Here's how the part is built. I have some questions about the finished solid (model axes, mm). Face numbers are marked on the shaded views. A direction names the side the tool comes from. Give positions to 0.01 mm unless a question says otherwise; leave off trailing zeros. Write each loop counter-clockwise with the first axis right and the second up, starting at its lowest first coordinate (ties: lowest second). Pieces come first, ordered by that corner, then holes. Notation, with made-up numbers: (-27.5, 53) -> (23.5, 53) arc R14 ccw to (23.5, 70) -> close; hole circle Ø3 at (82.5, 42). An arc over 180 degrees is marked (long way). Use one line per item in the form item = value.
```python
from build123d import *

# Parameters (mm, degrees)
SKETCH1_W           = 19
SKETCH1_H           = 19
BOSS_EXTRUDE1_DEPTH = 8
SKETCH2_R           = 1.75
CUT_EXTRUDE1_DEPTH  = 16.636495771
SKETCH3_W           = 6
SKETCH3_H           = 6
BOSS_EXTRUDE2_DEPTH = 12
FILLET1_R           = 2
SKETCH5_W           = 4
SKETCH5_H           = 4
BOSS_EXTRUDE4_DEPTH = 4
FILLET3_R           = 1


with BuildPart() as part:
    # Sketch1 → Boss-Extrude1 (new body)
    with BuildSketch(Plane(origin=(0, 0, 0), x_dir=(1, 0, 0), z_dir=(0, 1, 0))):
        Rectangle(SKETCH1_W, SKETCH1_H)
    extrude(amount=BOSS_EXTRUDE1_DEPTH)

    # Sketch2 → Cut-Extrude1 (cut, through all)
    with BuildSketch(Plane(origin=(0, 8, 0), x_dir=(1, 0, 0), z_dir=(0, 1, 0))):
        with Locations(Location((-6.5, 6.5, 0), (0, 0, 270))):
            Circle(SKETCH2_R)
        with Locations(Location((6.5, 6.5, 0), (0, 0, 270))):
            Circle(SKETCH2_R)
        with Locations(Location((-6.5, -6.5, 0), (0, 0, 270))):
            Circle(SKETCH2_R)
        with Locations(Location((6.5, -6.5, 0), (0, 0, 270))):
            Circle(SKETCH2_R)
    extrude(amount=-CUT_EXTRUDE1_DEPTH, mode=Mode.SUBTRACT)

    # Sketch3 → Boss-Extrude2 (add)
    with BuildSketch(Plane(origin=(0, 8, 0), x_dir=(1, 0, 0), z_dir=(0, 1, 0))):
        Rectangle(SKETCH3_W, SKETCH3_H)
    extrude(amount=BOSS_EXTRUDE2_DEPTH)

    # Fillet1
    fillet1_edges = [part.edges().sort_by_distance(p)[0] for p in [
        (-9.5, 4, -9.5),
        (9.5, 4, -9.5),
        (9.5, 4, 9.5),
        (-9.5, 4, 9.5),
    ]]
    fillet(fillet1_edges, radius=FILLET1_R)

    # Sketch5 → Boss-Extrude4 (add)
    with BuildSketch(Plane(origin=(0, 20, 0), x_dir=(1, 0, 0), z_dir=(0, 1, 0))):
        Rectangle(SKETCH5_W, SKETCH5_H)
    extrude(amount=BOSS_EXTRUDE4_DEPTH)

    # Fillet3
    fillet3_edges = [part.edges().sort_by_distance(p)[0] for p in [
        (-3, 8, 0),
        (-3, 14, -3),
        (0, 8, 3),
        (-3, 14, 3),
        (3, 8, 0),
        (3, 14, 3),
        (0, 8, -3),
        (3, 14, -3),
        (-2, 22, -2),
        (-2, 22, 2),
        (2, 22, 2),
        (2, 22, -2),
    ]]
    fillet(fillet3_edges, radius=FILLET3_R)


solid = part.part
```
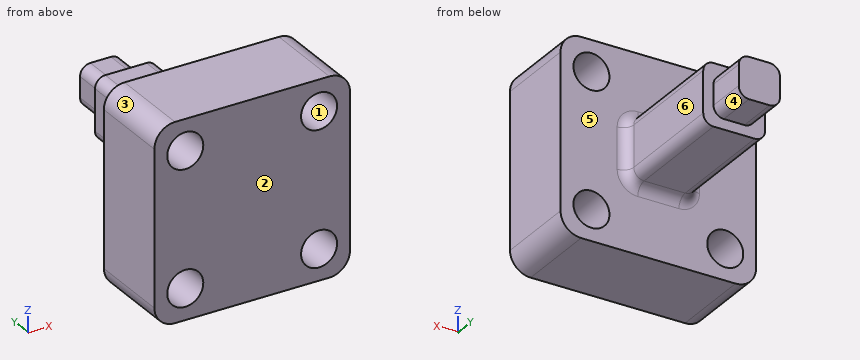
Q1. If we mould it in two halves opening along X, with no side actions, what happens to the marked faces 1, 2 and 3? For each: +X half, -X half, draft (parallel to the pull), parting line (faces both ways), or undercut.
Result set:
face_1 = undercut
face_2 = draft
face_3 = -X half
Q2. Will these pins go through, and if not, where does the flat tip stop? pin 1 Ø4.5 at (y, z) = (15, -0.5) entering from +X; pin 2 Ø2 at (y, z) = (21.5, 0) entering from -X; pin 3 Ø1.5 at (x, y) = (3.5, 19) entering from +Z; pin 4 Ø4 at (y, z) = (11.5, 7.5) entering from -X.
Result set:
pin_1 = 3
pin_2 = -2
pin_3 = 2.66
pin_4 = through
Q3. Which directions (+Z, -Z, +X, -X, +Y, -Y) give clear straight access to the entire face, cutting with the end or side of a thin tool? Please do the marked faces 4, 5 and 6.
Result set:
face_4 = -Z, +X, +Y
face_5 = +Y
face_6 = +Z, -Z, +X, +Y
Q4. I want a section at C-C, the plane y = 3.75. Write out the boundary of the cut face in (x, z), and give its area (3 significant figures).
Result set:
outline = (-9.5, -7.5) arc R2 ccw to (-7.5, -9.5) -> (7.5, -9.5) arc R2 ccw to (9.5, -7.5) -> (9.5, 7.5) arc R2 ccw to (7.5, 9.5) -> (-7.5, 9.5) arc R2 ccw to (-9.5, 7.5) -> close; hole circle Ø3.5 at (-6.5, -6.5); hole circle Ø3.5 at (-6.5, 6.5); hole circle Ø3.5 at (6.5, -6.5); hole circle Ø3.5 at (6.5, 6.5)
area = 319 mm2
Q5. I want a section at A-A, the plane x = 6.5. Write out the boundary of the cut face in (y, z), and give its area (3 significant figures).
Result set:
outline = (0, -9.5) -> (8, -9.5) -> (8, -8.25) -> (0, -8.25) -> close; (0, -4.75) -> (8, -4.75) -> (8, 4.75) -> (0, 4.75) -> close; (0, 8.25) -> (8, 8.25) -> (8, 9.5) -> (0, 9.5) -> close
area = 96.0 mm2
Q6. I want a section at D-D, the plane y = 11.75. Write out the boundary of the cut face in (x, z).
Result set:
outline = (-3, -2) arc R1 ccw to (-2, -3) -> (2, -3) arc R1 ccw to (3, -2) -> (3, 2) arc R1 ccw to (2, 3) -> (-2, 3) arc R1 ccw to (-3, 2) -> close
Q7. If I drill on line 1 along X through (y, z) = (5.25, -6.5); line 2 along Y through (x, z) = (-4, -1.25); line 3 along Y through (x, z) = (-1.75, -2.5), over which ranges is the centre line in solid material (lowest first)? Write a range as from..to.
Result set:
line_1 = -9.5..-8.25, -4.75..4.75, 8.25..9.5
line_2 = 0..8
line_3 = 0..20
Q8. I want a section at B-B, the plane z = -6.5. Write out the boundary of the cut face in (x, y), and give its area (3 significant figures).
Result set:
outline = (-9.5, 0) -> (-8.25, 0) -> (-8.25, 8) -> (-9.5, 8) -> close; (-4.75, 0) -> (4.75, 0) -> (4.75, 8) -> (-4.75, 8) -> close; (8.25, 0) -> (9.5, 0) -> (9.5, 8) -> (8.25, 8) -> close
area = 96.0 mm2
